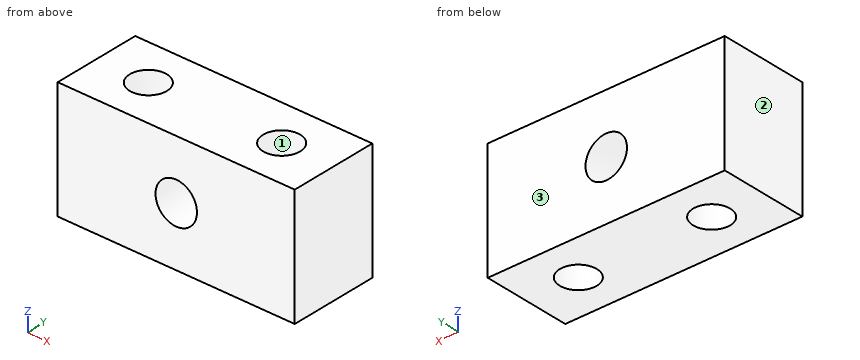
from build123d import *

# Parameters (mm, degrees)
SKETCH1_W           = 50.8
SKETCH1_H           = 19.05
SKETCH1_R           = 3.96875
BOSS_EXTRUDE1_DEPTH = 12.7
SKETCH2_R           = 4.445
CUT_EXTRUDE1_DEPTH  = 35.195796525


with BuildPart() as part:
    # Sketch1 → Boss-Extrude1 (new, symmetric)
    with BuildSketch(Plane.XY):
        Rectangle(SKETCH1_W, SKETCH1_H)
        with Locations(Location((-14.2875, 0, 0), (0, 0, 180))):
            Circle(SKETCH1_R, mode=Mode.SUBTRACT)
        with Locations(Location((14.2875, 0, 0), (0, 0, 180))):
            Circle(SKETCH1_R, mode=Mode.SUBTRACT)
    extrude(amount=BOSS_EXTRUDE1_DEPTH, both=True)

    # Sketch2 → Cut-Extrude1 (cut, through all)
    with BuildSketch(Plane(origin=(0, 9.525, 0), x_dir=(1, 0, 0), z_dir=(0, 1, 0))):
        with Locations(Location((0, 0, 0), (0, 0, 270))):
            Circle(SKETCH2_R)
    extrude(amount=-CUT_EXTRUDE1_DEPTH, mode=Mode.SUBTRACT)


solid = part.part
Check sheet for the modelled part. Datum: model origin and axes. Units: mm. Face numbers are marked on the shaded views. Give positions to 0.01 mm unless a question says otherwise; leave off trailing zeros. Loops run counter-clockwise (first coordinate to the right, second up) from the corner with the lowest first, then second, coordinate; pieces in that order, holes last. Notation, with made-up numbers: M 27,19 L 35,19 A21 ccw 35,54 Z; hole C -14.5,-33 d1. An arc over 180 degrees is marked long. Answer as a JSON object with one key per item and string values. Group by question number.
Q1. Cross-section at C-C on x = 0. Record the cut outline in (y, z) (3 decimals).
Q2. Release check for a two-part mould opening along X. For the marked faces 1, 2 and 3 record: released by +X, released by -X, zero draft, split by the parting line, or undercut.
Q3. Cross-section at A-A on y = -1. Record the cut outline in (x, z) (3 decimals).
Q4. Cross-section at D-D on y = 6. Record the cut outline in (x, z) (3 decimals).
Q5. Material ranges on line 1 along X through (y, z) = (1, 5); line 2 along Y through (x, z) = (14, -0.5) (3 decimals); line 3 along X through (y, z) = (2.5, 0) (3 decimals), recorded low to high. Write a range as [from, to].
Q6. Cross-section at B-B on z = 1.5. Record the cut outline in (x, y) (1 decimal), then the cut area to 3 significant figures.
Evaluation:
{
 "1": {"outline": "M -9.525,-12.7 L 9.525,-12.7 L 9.525,-4.445 L -9.525,-4.445 Z; M -9.525,4.445 L 9.525,4.445 L 9.525,12.7 L -9.525,12.7 Z"},
 "2": {"face 1": "undercut", "face 2": "released by -X", "face 3": "zero draft"},
 "3": {"outline": "M -25.4,-12.7 L -18.128,-12.7 L -18.128,12.7 L -25.4,12.7 Z; M -10.447,-12.7 L 10.447,-12.7 L 10.447,12.7 L -10.447,12.7 Z; M 18.128,-12.7 L 25.4,-12.7 L 25.4,12.7 L 18.128,12.7 Z; hole C 0,0 d8.89"},
 "4": {"outline": "M -25.4,-12.7 L 25.4,-12.7 L 25.4,12.7 L -25.4,12.7 Z; hole C 0,0 d8.89"},
 "5": {"line 1": "x = [-25.4, -18.13], [-10.45, 10.45], [18.13, 25.4]", "line 2": "y = [-9.525, -3.958], [3.958, 9.525]", "line 3": "x = [-25.4, -17.37], [-11.205, -4.445], [4.445, 11.205], [17.37, 25.4]"},
 "6": {"outline": "M -25.4,-9.5 L -4.2,-9.5 L -4.2,9.5 L -25.4,9.5 Z; M 4.2,-9.5 L 25.4,-9.5 L 25.4,9.5 L 4.2,9.5 Z; hole C -14.3,0 d7.9; hole C 14.3,0 d7.9", "area": "709 mm2"}
}
